Autodesk Inventor part; units mm, degrees
ref_plane "YZ Plane" through (0, 0, 0) normal (1, 0, 0) x (0, 1, 0)
ref_plane "XZ Plane" through (0, 0, 0) normal (0, 1, 0) x (-1, 0, 0)
ref_plane "XY Plane" through (0, 0, 0) normal (0, 0, 1) x (1, 0, 0)
sketch "스케치1" plane through (0, 0, 0) normal (0, 1, 0) x (-1, 0, 0)
  line L0 (8.1082, 12.9394) -> (-22.8918, 12.9394)
  line L1 (-24.8918, 10.9394) -> (-24.8918, -22.0606)
  line L2 (-24.8918, -22.0606) -> (10.1082, -22.0606)
  line L3 (10.1082, -22.0606) -> (10.1082, 10.9394)
  arc A0 (10.1082, 10.9394) -> (8.1082, 12.9394) centre (8.1082, 10.9394) ccw
  arc A1 (-22.8918, 12.9394) -> (-24.8918, 10.9394) centre (-22.8918, 10.9394) ccw
  line L4 (10.1082, -25.0606) -> (-24.8918, -25.0606)
  line L5 (10.1082, -22.0606) -> (10.1082, -25.0606)
  line L6 (-24.8918, -22.0606) -> (-24.8918, -25.0606)
  line L7 (-10.8918, -9.5606) -> (-10.8918, 0.4394)
  line L8 (-3.8918, -9.5606) -> (-3.8918, 0.4394)
  line L9 (-3.8918, 0.4394) -> (-10.8918, 0.4394)
  line L10 (-10.8918, -9.5606) -> (-3.8918, -9.5606)
  arc A2 (-10.8918, -9.5606) -> (-3.8918, -9.5606) centre (-7.3918, -9.5606) ccw
  arc A3 (-3.8918, 0.4394) -> (-10.8918, 0.4394) centre (-7.3918, 0.4394) ccw
  line L11 (-24.8918, 19.0606) -> (-24.8918, -10.9394)
  point P0 (0, 0)
  point P1 (-24.8918, 12.9394)
  point P2 (0, 0)
  point P3 (-3.8918, -4.5606)
  point P4 (-10.8918, -4.5606)
  point P5 (-7.3918, -23.5606)
  point P6 (-7.3918, -22.0606)
  point P7 (-7.3918, -13.0606)
  point P8 (-7.3918, 12.9394)
  point P9 (-7.3918, 3.9394)
  dimension "d0" = 35
  dimension "d1" = 35
  dimension "d2" = 2
  dimension "d3" = 2
  dimension "d14" = 3
  dimension "d20" = 10
  dimension "d21" = 7
  dimension "d22" = 14
  dimension "d23" = 14
  dimension "d24" = 14
  dimension "d26" = 9
extrude "돌출3" add sketch "스케치1" along normal blind 3 contours A0 L3 L2 L1 A1 L0 | L7 L9 L8 L10 | L10 A2 | A3 L9
extrude "돌출4" add sketch "스케치1" along normal blind 38 contours L5 L4 L6 L2
fillet "모깎기2" radius 2 4 edges at (24.8918, 38, -23.5606) (-10.1082, 38, -23.5606) (7.3918, 3, -22.0606) (7.3918, 0, -25.0606)
sketch "스케치6" plane through (24.8918, 2, -25.0606) normal (0, 0, -1) x (-1, 0, 0)
  line L0 (33, 36) -> (2, 36)
  line L1 (0, 34) -> (0, 1)
  line L2 (0, 1) -> (35, 1)
  line L3 (35, 1) -> (35, 34)
  arc A0 (35, 34) -> (33, 36) centre (33, 34) ccw
  arc A1 (2, 36) -> (0, 34) centre (2, 34) ccw
  line L4 (35, -2) -> (0, -2)
  line L5 (35, 1) -> (35, -2)
  line L6 (0, 1) -> (0, -2)
  line L7 (14, 13.5) -> (14, 23.5)
  line L8 (21, 13.5) -> (21, 23.5)
  line L9 (21, 23.5) -> (14, 23.5)
  line L10 (14, 13.5) -> (21, 13.5)
  arc A2 (14, 13.5) -> (21, 13.5) centre (17.5, 13.5) ccw
  arc A3 (21, 23.5) -> (14, 23.5) centre (17.5, 23.5) ccw
  line L11 (0, 42.063) -> (0, 12.063)
  line L12 (0, 0) -> (0, 34)
  line L13 (0, -2) -> (35, -2)
  point P0 (24.8918, -2)
  point P1 (24.6406, 23.0024)
  point P2 (0, 36)
  point P3 (24.6406, 23.0024)
  point P4 (14, 18.5)
  point P5 (21, 18.5)
  point P6 (17.2488, -0.5)
  point P7 (17.5, 1)
  point P8 (17.5, 10)
  point P9 (17.5, 36)
  point P10 (17.5, 27)
  dimension "d38" = 35
  dimension "d39" = 35
  dimension "d40" = 2
  dimension "d41" = 2
  dimension "d42" = 3
  dimension "d43" = 10
  dimension "d44" = 7
  dimension "d45" = 14
  dimension "d46" = 14
  dimension "d47" = 14
  dimension "d48" = 9
  dimension "d49" = 0
  dimension "d50" = 0
extrude "돌출5" cut sketch "스케치6" against normal blind 38 contours L7 L9 L8 L10 | L10 A2 | A3 L9
extrude "돌출6" cut sketch "스케치1" along normal blind 38 contours L7 L9 L8 L10 | L10 A2 | A3 L9
properties part number "L자 브라켓" material "강철, 합금"
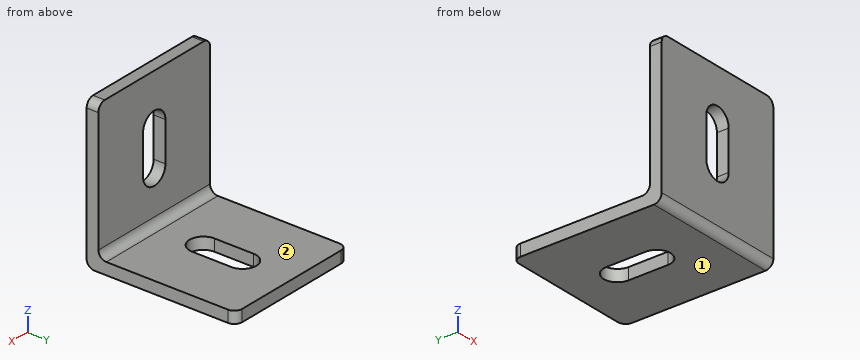
Check sheet for the modelled part. Datum: model origin and axes. Units: mm. Face numbers are marked on the shaded views. A direction names the side the tool comes from. Give positions to 0.01 mm unless a question says otherwise; leave off trailing zeros. Order: outer loops, then holes, each group sorted by start corner. A loop starts at its lowest first (then second) coordinate and runs counter-clockwise, first axis right, second up. Notation, with made-up numbers: (-22.5, 54) -> (12.5, 54) arc R12 cw to (12.5, 65) -> close; hole circle Ø10 at (10.5, 57.5). An arc over 180 degrees is marked (long way). Return JSON: item names as keys, results as strings.
1. Cross-section at B-B, the plane z = -1.5. Record the cut outline in (x, y), plus the area to 3 significant figures.
From the geometry:
{"outline": "(-10.11, 0) -> (3.89, 0) -> (3.89, 3) -> (-10.11, 3) -> close; (10.89, 0) -> (24.89, 0) -> (24.89, 3) -> (10.89, 3) -> close", "area": "84.0 mm^2"}
2. Cross-section at C-C, the plane x = 0. Record the cut outline in (y, z), plus the area to 3 significant figures.
From the geometry:
{"outline": "(0, -23.06) arc R2 ccw to (2, -25.06) -> (38, -25.06) -> (38, -22.06) -> (5, -22.06) arc R2 cw to (3, -20.06) -> (3, 12.94) -> (0, 12.94) -> close", "area": "219 mm^2"}
3. Set-up check for the marked faces 1 and 2: record each of +Z, -Z, +X, -X, +Y, -Y from which the full face is reachable in a straight line by a thin tool's end or side.
From the geometry:
{"face 1": "-Z, +X, -X, +Y, -Y", "face 2": "+Z, +X, -X, +Y"}
4. Material ranges on probe 1 along Y at (x, z) = (-3, -12); probe 2 along Z at (x, y) = (22.5, 30); probe 3 along Y at (x, z) = (19, -21), recorded low to high. Write a range as [from, to].
From the geometry:
{"probe 1": "[0, 3]", "probe 2": "[-25.06, -22.06]", "probe 3": "[0, 3.23]"}
5. Go/stop test with flat-tipped pins: P1, Ø4, axis at x = 7, z = -1, coming from the +Y side; P2, Ø8, axis at x = 7, z = 4, coming from the +Y side; P3, Ø10, axis at x = 3, y = 25, coming from the +Z side. Record where each tip stops, or that it passes through.
From the geometry:
{"P1": "through", "P2": "y = 3", "P3": "z = -22.06"}
6. Cross-section at A-A, the plane x = 6. Record the cut outline in (y, z), plus the area to 3 significant figures.
From the geometry:
{"outline": "(0, -23.06) arc R2 ccw to (2, -25.06) -> (12.29, -25.06) -> (12.29, -22.06) -> (5, -22.06) arc R2 cw to (3, -20.06) -> (3, -12.77) -> (0, -12.77) -> close; (0, 3.65) -> (3, 3.65) -> (3, 12.94) -> (0, 12.94) -> close; (28.71, -25.06) -> (38, -25.06) -> (38, -22.06) -> (28.71, -22.06) -> close", "area": "120 mm^2"}
7. Cross-section at D-D, the plane y = 28. Record the cut outline in (x, z).
From the geometry:
{"outline": "(-10.11, -25.06) -> (4.94, -25.06) -> (4.94, -22.06) -> (-10.11, -22.06) -> close; (9.84, -25.06) -> (24.89, -25.06) -> (24.89, -22.06) -> (9.84, -22.06) -> close"}
